from build123d import *
from build123d.topology import SkipClean

# Parameters (mm, degrees)
BOSS_EXTRUDE1_DEPTH = 30
CUT_EXTRUDE1_START  = -20
SKETCH2_R           = 10
SKETCH2_R_2         = 5
CUT_EXTRUDE1_DEPTH  = 10


with BuildPart() as part:
    # Sketch1 → Boss-Extrude1 (new body)
    with BuildSketch(Plane.XY):
        with BuildLine():
            ThreePointArc((2, 4.582575695), (0, 5), (-2, 4.582575695))
            Line((-2, 4.582575695), (-2, 3))
            Line((-2, 3), (2, 3))
            Line((2, 3), (2, 4.582575695))
        make_face()
        with BuildLine():
            Line((-2, 3), (-2, 4.582575695))
            ThreePointArc((-2, 4.582575695), (-2.738612788, -4.183300133), (5, 0))
            ThreePointArc((5, 0), (4.183300133, 2.738612788), (2, 4.582575695))
            Line((2, 4.582575695), (2, 3))
            Line((2, 3), (-2, 3))
        make_face()
        with BuildLine():
            Line((2, 7), (-2, 7))
            Line((-2, 7), (-2, 4.582575695))
            ThreePointArc((-2, 4.582575695), (0, 5), (2, 4.582575695))
            Line((2, 4.582575695), (2, 7))
        make_face()
    extrude(amount=BOSS_EXTRUDE1_DEPTH)

    # Sketch2 → Cut-Extrude1 (cut)
    with SkipClean():  # the faces are left unmerged after this step: merging them gives an invalid solid
        with BuildSketch(Plane.XY.offset(30).offset(CUT_EXTRUDE1_START)):
            Circle(SKETCH2_R)
            with Locations(Location((0, 0, 0), (0, 0, 113.578178478))):
                Circle(SKETCH2_R_2, mode=Mode.SUBTRACT)
        extrude(amount=CUT_EXTRUDE1_DEPTH, mode=Mode.SUBTRACT)


solid = part.part
Work out the finished part from the listing and answer in its coordinate system (mm). A direction names the side the tool comes from. Give positions to 0.01 mm unless a question says otherwise; leave off trailing zeros. Loops run counter-clockwise (first coordinate to the right, second up) from the corner with the lowest first, then second, coordinate; pieces in that order, holes last. Notation, with made-up numbers: (28, 57.5) - (40, 57.5) arc R21 cw to (40, 85.5) - close; hole circle Ø8 at (63.25, 39). An arc over 180 degrees is marked (long way). Answer in a Markdown table with one row per item. Add a question column.
Q1. A tool of negligible diameter and unlimited length cuts with its end or side. For faces 1 (the flat face through (-2, 6, 5)), 2 (the flat face through (2, 6, 25)), 3 (the flat face through (0, 1, 0)), from which of +Z, -Z, +X, -X, +Y, -Y can it reach the whole face along a straight path? Write none if from no direction.
Q2. Consider line 1 along Z through (x, y) = (0, 6.25); line 2 along X through (y, z) = (5.5, 22.25); line 3 along Y through (x, z) = (2.75, 27.25). Determine where each line is inside the solid, lowest interval first.
Q3. The part is cut by section A-A (y = 6.25). Determine the outline of the cut face in (x, z), and give its area (3 significant figures).
Q4. The part is cut by section C-C (x = 0). Determine the outline of the cut face in (y, z), and give its area (3 significant figures).
Q5. The part is cut by section D-D (y = 4). Determine the outline of the cut face in (x, z), and give its area (3 significant figures).
Q6. Each of these flat-tipped pins is pushed along its axis until it touches: P1, Ø4, axis at y = 4, z = 12.5, coming from the +X side; P2, Ø2.5, axis at y = 6, z = 25, coming from the +X side; P3, Ø1.2, axis at y = 6, z = 25, coming from the -X side. Where does it stop, or does it pass through?
Q7. The part is cut by section B-B (z = 9.5). Determine the outline of the cut face in (x, y), and give its area (3 significant figures).
Solution:
| question | item | result |
|---|---|---|
| 1 | face 1 | +Z, -Z, -X, +Y |
| 1 | face 2 | +Z, -Z, +X, +Y |
| 1 | face 3 | -Z, +X, -X, +Y, -Y |
| 2 | line 1 | z = 0 to 10, 20 to 30 |
| 2 | line 2 | x = -2 to 2 |
| 2 | line 3 | y = -4.18 to 4.18 |
| 3 | outline | (-2, 0) - (2, 0) - (2, 10) - (-2, 10) - close; (-2, 20) - (2, 20) - (2, 30) - (-2, 30) - close |
| 3 | area | 80.0 mm² |
| 4 | outline | (-5, 0) - (7, 0) - (7, 10) - (5, 10) - (5, 20) - (7, 20) - (7, 30) - (-5, 30) - close |
| 4 | area | 340 mm² |
| 5 | outline | (-3, 0) - (3, 0) - (3, 30) - (-3, 30) - close |
| 5 | area | 180 mm² |
| 6 | P1 | stops at x = 4.58 |
| 6 | P2 | stops at x = 2 |
| 6 | P3 | stops at x = -2 |
| 7 | outline | (-2, 4.58) arc R5 ccw (long way) to (2, 4.58) - (2, 7) - (-2, 7) - close |
| 7 | area | 87.1 mm² |
